Input: dimensioned drawing with shaded views. Units: mm. Origin: part minimum x, y, z. A direction names the side the tool comes from. Give positions to 0.01 mm unless a question says otherwise; leave off trailing zeros. Loops run counter-clockwise (first coordinate to the right, second up) from the corner with the lowest first, then second, coordinate; pieces in that order, holes last. Notation, with made-up numbers: M 75.5,71.5 L 83.5,71.5 A31 cw 83.5,95.5 Z; hole C 34.5,85.25 d7. An arc over 180 degrees is marked long. Answer in a Markdown table with one row per item.
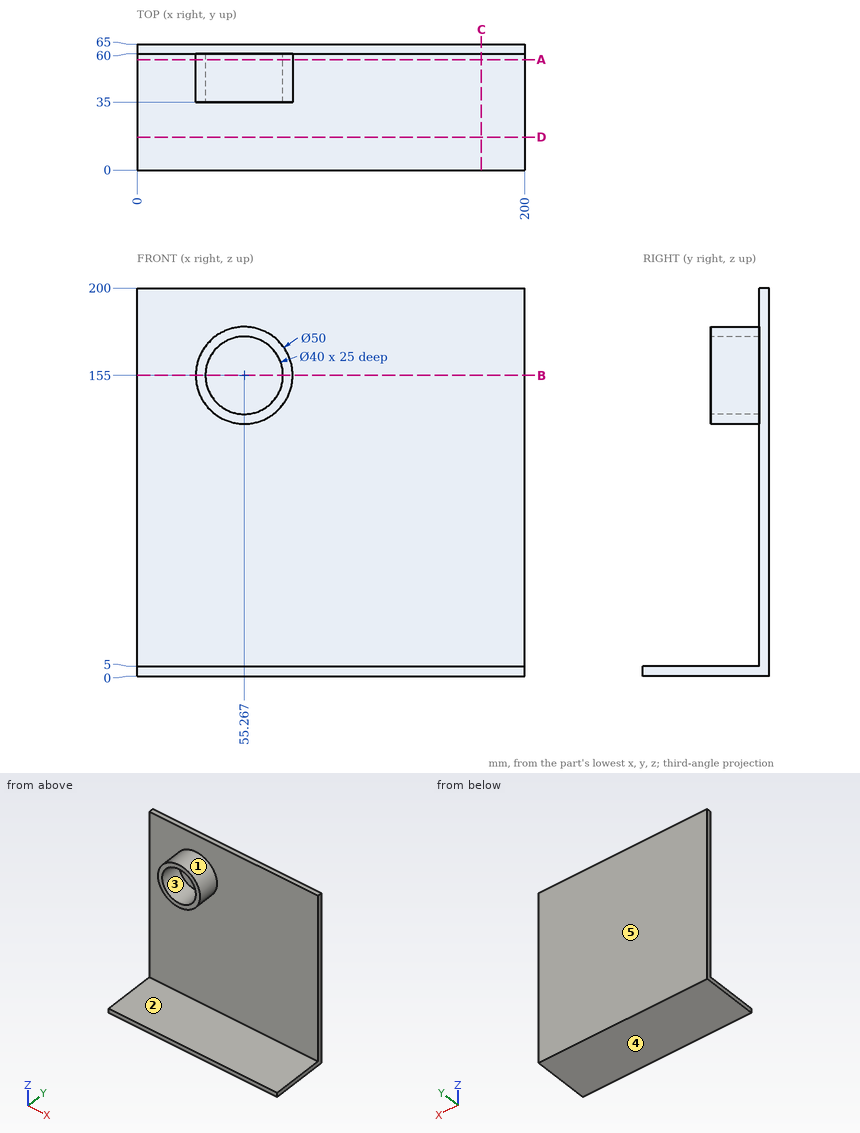
Q1. Reachability of the marked faces 1 and 2 from +Z, -Z, +X, -X, +Y, -Y: full face, straight path, thin tool, end or side. Return the list, or none.
Values follow:
| item | result |
|---|---|
| face 1 | -Y |
| face 2 | +X, -X, -Y |
Q2. Section query C-C (x = 177.5). Output: boundary loops of the cut face in (y, z).
Values follow:
| item | result |
|---|---|
| outline | M 0,0 L 65,0 L 65,200 L 60,200 L 60,5 L 0,5 Z |
Q3. Mould query, pull axis Z, two halves, no side actions, for the marked faces 3, 4 and 5. Classes: +Z half, -Z half, draft (parallel to the pull), parting line (faces both ways), or undercut.
Values follow:
| item | result |
|---|---|
| face 3 | undercut |
| face 4 | -Z half |
| face 5 | draft |
Q4. Ray query, probe 1 along Z at (x, y) = (54, 51); probe 2 along Z at (x, y) = (178.5, 58); probe 3 along Z at (x, y) = (46.5, 45) (1 decimal). Return the intervals inside material, ascending. Write a range as from..to.
Values follow:
| item | result |
|---|---|
| probe 1 | 0..5, 130.03..135.04, 174.96..179.97 |
| probe 2 | 0..5 |
| probe 3 | 0..5, 131.6..137, 173..178.4 |
Q5. Contact query for flat-ended pins moving along their axis: pin 1 Ø1 at (y, z) = (54.5, 135) entering from +X; pin 2 Ø25 at (x, z) = (50.5, 150.5) entering from -Y; pin 3 Ø1 at (x, y) = (34.5, 53.5) entering from +Z. Output: stop coordinate, or through.
Values follow:
| item | result |
|---|---|
| pin 1 | x = 70.91 |
| pin 2 | y = 60 |
| pin 3 | z = 169.64 |
Q6. Section query A-A (y = 57). Output: boundary loops of the cut face in (x, z).
Values follow:
| item | result |
|---|---|
| outline | M 0,0 L 200,0 L 200,5 L 0,5 Z; C 55.27,155 d50; hole C 55.27,155 d40 |
Q7. Section query B-B (z = 155). Output: boundary loops of the cut face in (x, y).
Values follow:
| item | result |
|---|---|
| outline | M 0,60 L 30.27,60 L 30.27,35 L 35.27,35 L 35.27,60 L 75.27,60 L 75.27,35 L 80.27,35 L 80.27,60 L 200,60 L 200,65 L 0,65 Z |
Q8. Section query D-D (y = 17). Output: boundary loops of the cut face in (x, z).
Values follow:
| item | result |
|---|---|
| outline | M 0,0 L 200,0 L 200,5 L 0,5 Z |
